Solid Edge part; units mm, degrees
sketch "Sketch1" plane through (0, 0, 0) normal (0, 0, 1) x (1, 0, 0)
  circle A0 centre (-13.4214, 4.1158) radius 7.5
  line L0 (-103.4214, 174.1158) -> (-28.4214, 14.1158)
  line L1 (-28.4214, 14.1158) -> (-28.4214, -5.8842)
  line L2 (-28.4214, -5.8842) -> (-85.1518, -195.8842)
  line L3 (-85.1518, -195.8842) -> (-55.1518, -195.8842)
  line L4 (-55.1518, -195.8842) -> (1.5786, -5.8842)
  line L5 (1.5786, 14.1158) -> (1.5786, -5.8842)
  line L6 (-73.4214, 174.1158) -> (1.5786, 14.1158)
  line L7 (-73.4214, 234.1158) -> (-73.4214, 174.1158)
  line L8 (-103.4214, 234.1158) -> (-73.4214, 234.1158)
  line L9 (-103.4214, 174.1158) -> (-103.4214, 234.1158)
  dimension "D1" = 28.4214
  dimension "D2" = 103.4214
  dimension "D3" = 103.4214
  dimension "D4" = 73.4214
  dimension "D5" = 1.5786
  dimension "D6" = 13.4214
extrude "Protrusion1" add sketch "Sketch1" along normal blind 20
Could you check a few things on this model? Use its own coordinates, in mm. A direction names the side the tool comes from. Give positions to 0.01 mm unless a question says otherwise; leave off trailing zeros. Order: outer loops, then holes, each group sorted by start corner. A loop starts at its lowest first (then second) coordinate and runs counter-clockwise, first axis right, second up. Notation, with made-up numbers: (77, 50.5) -> (130, 50.5) arc R29 cw to (130, 74.5) -> close; hole circle Ø7 at (80.5, 26). An arc over 180 degrees is marked (long way). Return JSON: item names as keys, results as strings.
1. Imagine slicing it at C-C on x = -59.5. List the corners of the cut face in (y, z) for me.
Answer list:
{"outline": "(-195.88, 0) -> (-109.97, 0) -> (-109.97, 20) -> (-195.88, 20) -> close; (80.42, 0) -> (144.42, 0) -> (144.42, 20) -> (80.42, 20) -> close"}
2. Imagine slicing it at B-B on z = 14.25. List the corners of the cut face in (x, y) for me.
Answer list:
{"outline": "(-103.42, 174.12) -> (-28.42, 14.12) -> (-28.42, -5.88) -> (-85.15, -195.88) -> (-55.15, -195.88) -> (1.58, -5.88) -> (1.58, 14.12) -> (-73.42, 174.12) -> (-73.42, 234.12) -> (-103.42, 234.12) -> close; hole circle Ø15 at (-13.42, 4.12)"}
3. On a 3-axis mill with a long thin cutter (end or side, diameter ignored), from which of +Z, -Z, +X, -X, +Y, -Y can I reach the whole of each face in a straight line? I mean faces 5 (the flat face through (-36, 36, 20)), 6 (the flat face through (-56.39, -99.55, 9.86)), 7 (the flat face through (-73.421, 205, 10)). Say none if no direction works.
Answer list:
{"face 5": "+Z, +X, -X, +Y, -Y", "face 6": "+Z, -Z, -X", "face 7": "+Z, -Z, +X, +Y"}
4. Imagine slicing it at A-A on x = -11. List the corners of the cut face in (y, z) for me.
Answer list:
{"outline": "(-48.01, 0) -> (-2.98, 0) -> (-2.98, 20) -> (-48.01, 20) -> close; (11.21, 0) -> (40.95, 0) -> (40.95, 20) -> (11.21, 20) -> close"}
5. For pin 1 Ø3 at (x, z) = (-65, 11) entering from +Y; pin 2 Ø5 at (y, z) = (-79, 6.5) entering from -X; pin 3 Ø3 at (y, z) = (-45.5, 3) entering from +X, each with a flat end and sliding along its axis, tell me the tip position at first contact or that it passes through.
Answer list:
{"pin 1": "stops at y = 159.35", "pin 2": "stops at x = -51", "pin 3": "stops at x = -9.8"}
6. Imagine slicing it at D-D on y = -54. List the corners of the cut face in (x, z) for me.
Answer list:
{"outline": "(-42.79, 0) -> (-12.79, 0) -> (-12.79, 20) -> (-42.79, 20) -> close"}
7. I need wall thicknesses on line 1 (X direction, y = 130, z = 4.5); line 2 (X direction, y = 54, z = 3.5); line 3 (Y direction, x = -97.5, z = 8.5). Which ranges of each line are inside material? Lowest first, please. Write a range as from..to.
Answer list:
{"line 1": "x = -82.74..-52.74", "line 2": "x = -47.12..-17.12", "line 3": "y = 161.48..234.12"}
8. Thinking about a two-plate mould opening in Y: for faces 1 (the flat face through (-70, -195.884, 10)), 2 (the flat face through (-36.45, 95.24, 9.86)), 3 (the flat face through (-28.421, 4, 10)), 4 (the flat face through (-66.45, 95.24, 9.86)), which applies, pulls with the +Y half, pulls with the -Y half, needs draft (parallel to the pull), parting line crosses it, or undercut?
Answer list:
{"face 1": "pulls with the -Y half", "face 2": "pulls with the +Y half", "face 3": "undercut", "face 4": "undercut"}
